Part model, mm, in its own coordinate system. A direction names the side the tool comes from. Give positions to 0.01 mm unless a question says otherwise; leave off trailing zeros. Write each loop counter-clockwise with the first axis right and the second up, starting at its lowest first coordinate (ties: lowest second). Pieces come first, ordered by that corner, then holes.
```python
from build123d import *

# Parameters (mm, degrees)
F0_R     = 10.85
F1_DEPTH = 8
F2_R     = 11.047434
F3_DEPTH = 25
F4_R     = 2
F5_R     = 2.5
F6_DEPTH = 25


with BuildPart() as f1:
    # F0 (on Front) → F1 (new body)
    with BuildSketch(Plane.XZ):
        with BuildLine():
            Line((-40.454113, 50.402456), (-40.454113, 69.742202))
            ThreePointArc((-40.454113, 69.742202), (-55.454113, 84.742202), (-70.454113, 69.742202))
            Line((-70.454113, 69.742202), (-70.454113, 50.402456))
            Line((-70.454113, 50.402456), (-87.202824, 40.732583))
            ThreePointArc((-87.202824, 40.732583), (-92.693205, 20.242202), (-72.202824, 14.751821))
            Line((-72.202824, 14.751821), (-55.454113, 24.421694))
            Line((-55.454113, 24.421694), (-38.705401, 14.751821))
            ThreePointArc((-38.705401, 14.751821), (-18.21502, 20.242202), (-23.705401, 40.732583))
            Line((-23.705401, 40.732583), (-40.454113, 50.402456))
        make_face()
        Polygon((-71.402824, 32.534209), (-71.402824, 22.950195), (-79.702824, 18.158187), (-88.002824, 22.950195), (-88.002824, 32.534209), (-79.702824, 37.326216), align=None, mode=Mode.SUBTRACT)
        Polygon((-39.505401, 32.534209), (-31.205401, 37.326216), (-22.905401, 32.534209), (-22.905401, 22.950195), (-31.205401, 18.158187), (-39.505401, 22.950195), align=None, mode=Mode.SUBTRACT)
        with Locations((-55.454113, 41.742202)):
            Circle(F0_R, mode=Mode.SUBTRACT)
        Polygon((-55.454113, 79.326216), (-47.154113, 74.534209), (-47.154113, 64.950195), (-55.454113, 60.158187), (-63.754113, 64.950195), (-63.754113, 74.534209), align=None, mode=Mode.SUBTRACT)
    extrude(amount=F1_DEPTH)

    # F2 (on face) → F3 (join)
    with BuildSketch(Plane.XZ.offset(8)):
        with Locations((-55.454113, 69.742202)):
            Circle(F2_R)
    extrude(amount=F3_DEPTH)

    # F4
    f4_edges = [f1.edges().sort_by_distance(p)[0] for p in [
        (-66.501547, -33, 69.742202),
    ]]
    fillet(f4_edges, radius=F4_R)

    # F5 (on face) → F6 (cut)
    with BuildSketch(Plane.XZ.offset(33)):
        with Locations((-55.454113, 69.742202)):
            Circle(F5_R)
    extrude(amount=-F6_DEPTH, mode=Mode.SUBTRACT)


solid = f1.part
```
1) Saw through at C-C, the plane z = 46. Write the cut outline in (x, y).
Answers follow:
outline: (-78.08, -8) - (-65.43, -8) - (-65.43, 0) - (-78.08, 0) - close; (-45.47, -8) - (-32.83, -8) - (-32.83, 0) - (-45.47, 0) - close
2) Wall check: L1, parallel to X at y = -11, z = 70; L2, parallel to Y at x = -49, z = 55; L3, parallel to Z at x = -57, y = -3.5. Give the ranges that are in metal, low to high.
Answers follow:
L1: x = -66.5 to -57.94, -52.97 to -44.41
L2: y = -8 to 0
L3: z = 23.53 to 31, 52.48 to 61.05, 78.43 to 84.66
3) Saw through at D-D, the plane y = -6. Write the cut outline in (x, z).
Answers follow:
outline: (-87.2, 40.73) arc R15 ccw to (-72.2, 14.75) - (-55.45, 24.42) - (-38.71, 14.75) arc R15 ccw to (-23.71, 40.73) - (-40.45, 50.4) - (-40.45, 69.74) arc R15 ccw to (-70.45, 69.74) - (-70.45, 50.4) - close; hole (-88, 22.95) - (-79.7, 18.16) - (-71.4, 22.95) - (-71.4, 32.53) - (-79.7, 37.33) - (-88, 32.53) - close; hole circle Ø21.7 at (-55.45, 41.74); hole (-63.75, 64.95) - (-55.45, 60.16) - (-47.15, 64.95) - (-47.15, 74.53) - (-55.45, 79.33) - (-63.75, 74.53) - close; hole (-39.51, 22.95) - (-31.21, 18.16) - (-22.91, 22.95) - (-22.91, 32.53) - (-31.21, 37.33) - (-39.51, 32.53) - close
4) 3-axis set-ups, long thin cutter, end or side, ignore diameter. For faces 4 (the face through (-51.362, -3.944, 76.964)), 5 (the face through (-56.892, -19.339, 80.696)), 6 (the face through (-70.454, -4, 60)), 7 (the face through (-71.403, -4, 28)): which of +Z, -Z, +X, -X, +Y, -Y reach the whole face in a straight line?
Answers follow:
face 4: +Y
face 5: -Y
face 6: +Z, -X, +Y, -Y
face 7: +Y, -Y
5) Saw through at A-A, the plane z = 27.5. Write the cut outline in (x, y), then the cut area to 3 significant figures.
Answers follow:
outline: (-94.7, -8) - (-88, -8) - (-88, 0) - (-94.7, 0) - close; (-71.4, -8) - (-39.51, -8) - (-39.51, 0) - (-71.4, 0) - close; (-22.91, -8) - (-16.21, -8) - (-16.21, 0) - (-22.91, 0) - close
area: 362 mm2
6) Two-plate mould, pull along Z, no slides. Class faces 1 (the face through (-55.78, -20.68, 72.22)), 2 (the face through (-18.38, -3.94, 19.96)), 3 (the face through (-40.454, -4, 60)): +Z half, -Z half, draft (parallel to the pull), parting line (faces both ways), or undercut.
Answers follow:
face 1: undercut
face 2: parting line
face 3: draft
7) Saw through at B-B, the plane x = -81. Write the cut outline in (y, z), then the cut area to 3 significant figures.
Answers follow:
outline: (-8, 12.8) - (0, 12.8) - (0, 18.91) - (-8, 18.91) - close; (-8, 36.58) - (0, 36.58) - (0, 44.31) - (-8, 44.31) - close
area: 111 mm2
8) Pin check, flat tips, straight feed: pin 1 Ø4 at (y, z) = (-3, 70.5) entering from +X; pin 2 Ø5 at (x, z) = (-54.5, 66) entering from +Y; pin 3 Ø3 at (x, z) = (-55.45, 69.74) entering from -Y; pin 4 Ø2.5 at (y, z) = (-3, 57.5) entering from -X. Stop position of each tip, or through.
Answers follow:
pin 1: stops at x = -40.45
pin 2: stops at y = -8
pin 3: passes through
pin 4: stops at x = -70.45
